Autodesk Inventor part; units mm, degrees
ref_plane "YZ Plane" through (0, 0, 0) normal (1, 0, 0) x (0, 1, 0)
ref_plane "XZ Plane" through (0, 0, 0) normal (0, 1, 0) x (-1, 0, 0)
ref_plane "XY Plane" through (0, 0, 0) normal (0, 0, 1) x (1, 0, 0)
sketch "Sketch1" plane through (0, 0, 0) normal (0, 1, 0) x (-1, 0, 0)
  line L0 (0, 0) -> (300, 0)
  line L1 (300, 0) -> (300, -300)
  line L2 (300, -300) -> (0, -300)
  line L3 (0, -300) -> (0, 0)
  dimension "d0" = 300
  dimension "d1" = 300
extrude "Extrusion1" add sketch "Sketch1" along normal blind 300
sketch "Sketch3" plane through (0, 0, 0) normal (0, -1, 0) x (1, 0, 0)
  line L0 (-10, -270) -> (-280, -270)
  line L1 (-280, -270) -> (-280, -30)
  line L2 (-280, -30) -> (-10, -30)
  line L3 (-10, -30) -> (-10, -270)
  line L4 (0, 0) -> (0, -300)
  line L5 (-300, -300) -> (-300, 0)
  line L6 (0, -300) -> (-300, -300)
  line L7 (-300, 0) -> (0, 0)
  dimension "d10" = 10
  dimension "d11" = 20
  dimension "d12" = 30
  dimension "d13" = 30
extrude "Extrusion3" cut sketch "Sketch3" against normal blind 10 contours L0 L1 L2 L3
sketch "Sketch5" plane through (-300, 0, -300) normal (-1, 0, 0) x (0, 0, 1)
  line L0 (10, 10) -> (290, 10)
  line L1 (290, 10) -> (290, 290)
  line L2 (290, 290) -> (10, 290)
  line L3 (10, 290) -> (10, 10)
  line L4 (0, 300) -> (300, 300)
  line L5 (0, 0) -> (300, 0)
  line L6 (0, 0) -> (0, 300)
  line L7 (300, 0) -> (300, 300)
  dimension "d22" = 10
  dimension "d23" = 10
  dimension "d24" = 10
  dimension "d25" = 10
extrude "Extrusion5" cut sketch "Sketch5" against normal blind 290 contours L3 L2 L1 L0
sketch "Sketch7" plane through (0, 0, 0) normal (1, 0, 0) x (0, 0, -1)
  circle A0 centre (150, 150) radius 2.5
  line L0 (0, 300) -> (300, 300)
  line L1 (300, 0) -> (300, 300)
  point P0 (0, 0)
  dimension "d37" = 5
  dimension "d38" = 150
  dimension "d39" = 150
extrude "Extrusion7" cut sketch "Sketch7" against normal blind 10
sketch "Sketch8" plane through (0, 300, 0) normal (0, 1, 0) x (1, 0, 0)
  circle A0 centre (-150, 150) radius 7.5
  line L0 (0, 0) -> (0, 300)
  line L1 (0, 300) -> (-300, 300)
  dimension "d42" = 15
  dimension "d43" = 150
  dimension "d44" = 150
extrude "Extrusion8" cut sketch "Sketch8" against normal through all
properties part number "temporary" material "PC/ABS Plastic"
Part model, mm, in its own coordinate system. A direction names the side the tool comes from. Coordinates: 2 decimals unless noted, no trailing zeros. Loops run counter-clockwise (first coordinate to the right, second up) from the corner with the lowest first, then second, coordinate; pieces in that order, holes last. Notation, with made-up numbers: M 75.25,-38.75 L 82.25,-38.75 A19 cw 82.25,-18.75 Z; hole C -34.5,2.5 d11. An arc over 180 degrees is marked long. Use a Markdown table: item, result. Add a question column.
Q1. Mould opens along Z. For faces 4 (the flat face through (-147, 5, -30)), 5 (the flat face through (-152, 148, -300)), 6 (the flat face through (-10, 143, -148)), 7 (the flat face through (-148, 300, -181)) say: +Z half, -Z half, draft (parallel to the pull), parting line (faces both ways), or undercut.
Q2. Cut at B-B (z = -69). Write the cut outline in (x, y), and give its area (3 significant figures).
Q3. Probe L1, parallel to Y at x = -282, z = -142.5; L2, parallel to Z at x = -133, y = 193; L3, parallel to Y at x = -5.5, z = -150. List the from-to ranges inside material, lowest first.
Q4. Cut at A-A (x = -150). Write the cut outline in (y, z), and give its area (3 significant figures).
Q5. Which spindle directions (+Z, -Z, +X, -X, +Y, -Y) get a long thin tool onto all of the face, cutting with end or side? Do faces 1 (the flat face through (-280, 5, -152)), 2 (the flat face through (-285, 10, -171)), 3 (the flat face through (-160, 0, -27)). Say none if no direction does.
Q6. Pin check, flat tips, straight feed: P1, Ø12, axis at y = 78, z = -186.5, coming from the +X side; P2, Ø10, axis at y = 198.5, z = -209.5, coming from the -X side; P3, Ø1, axis at x = -155.5, z = -103.5, coming from the -Y side. Stop position of each tip, or through.
Q7. Cut at C-C (y = 26). Write the cut outline in (x, z), and give its area (3 significant figures).
Q8. Cut at D-D (x = -33). Write the cut outline in (y, z), and give its area (3 significant figures).
Worked out:
| question | item | result |
|---|---|---|
| 1 | face 4 | undercut |
| 1 | face 5 | -Z half |
| 1 | face 6 | undercut |
| 1 | face 7 | draft |
| 2 | outline | M -300,0 L -280,0 L -280,10 L -300,10 Z; M -300,290 L -10,290 L -10,0 L 0,0 L 0,300 L -300,300 Z |
| 2 | area | 6,100 mm2 |
| 3 | L1 | y = 0 to 10, 290 to 300 |
| 3 | L2 | z = -300 to -290, -10 to 0 |
| 3 | L3 | y = 0 to 147.5, 152.5 to 300 |
| 4 | outline | M 0,-300 L 300,-300 L 300,-157.5 L 290,-157.5 L 290,-290 L 10,-290 L 10,-270 L 0,-270 Z; M 0,-30 L 10,-30 L 10,-10 L 290,-10 L 290,-142.5 L 300,-142.5 L 300,0 L 0,0 Z |
| 4 | area | 9,050 mm2 |
| 5 | face 1 | -Y |
| 5 | face 2 | -X |
| 5 | face 3 | +Z, -Z, +X, -X, -Y |
| 6 | P1 | stops at x = 0 |
| 6 | P2 | stops at x = -10 |
| 6 | P3 | stops at y = 290 |
| 7 | outline | M -300,-300 L 0,-300 L 0,0 L -300,0 L -300,-10 L -10,-10 L -10,-290 L -300,-290 Z |
| 7 | area | 8,800 mm2 |
| 8 | outline | M 0,-300 L 300,-300 L 300,0 L 0,0 L 0,-30 L 10,-30 L 10,-10 L 290,-10 L 290,-290 L 10,-290 L 10,-270 L 0,-270 Z |
| 8 | area | 9,200 mm2 |
